Read the model definition and answer for the solid it produces. Units are mm, in the model's axes. Face numbers are marked on the shaded views. A direction names the side the tool comes from. Coordinates: 2 decimals unless noted, no trailing zeros. Loops run counter-clockwise (first coordinate to the right, second up) from the corner with the lowest first, then second, coordinate; pieces in that order, holes last. Notation, with made-up numbers: M 33.5,21 L 51.5,21 A8 ccw 51.5,36 Z; hole C -2.75,28.5 d8. An arc over 180 degrees is marked long. One line per item, written item: value. Start each with the question number.
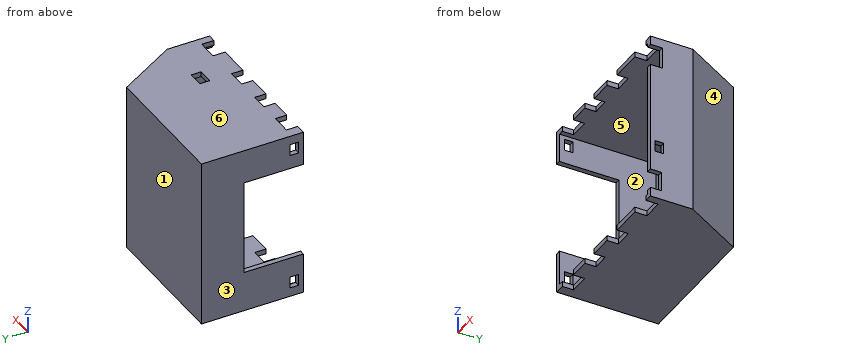
```python
from build123d import *

# Parameters (mm, degrees)
BOSS_EXTRUDE1_DEPTH = 100
SHELL1_T            = -3
SKETCH2_W           = 56.015644735
SKETCH2_H           = 35
CUT_EXTRUDE1_DEPTH  = 10
SKETCH3_W           = 12.606592538
SKETCH3_H           = 6.980178381
SKETCH3_W_2         = 11.515112664
SKETCH3_H_2         = 6.37986445
CUT_EXTRUDE2_DEPTH  = 10
SKETCH4_W           = 9.169229256
SKETCH4_H           = 5.894504522
CUT_EXTRUDE3_DEPTH  = 10
SKETCH5_W           = 6.776014824
SKETCH5_H           = 5.054240566
CUT_EXTRUDE4_DEPTH  = 10
SKETCH6_W           = 11.990530565
SKETCH6_H           = 7.12730724
CUT_EXTRUDE5_DEPTH  = 122.475306133
SKETCH8_W           = 6.563036955
SKETCH8_H           = 5.005706152
CUT_EXTRUDE6_DEPTH  = 10
SKETCH9_W           = 11.789009043
SKETCH9_H           = 6.673883815
SKETCH9_W_2         = 10.731021053
SKETCH9_H_2         = 6.623503435
SKETCH9_W_3         = 9.824174203
SKETCH9_H_3         = 6.573123054
CUT_EXTRUDE7_DEPTH  = 122.475306133


with BuildPart() as part:
    # Sketch1 → Boss-Extrude1 (new body)
    with BuildSketch(Plane.XY):
        Polygon((-50, 12.5), (-50, 47.5), (29.792740578, 47.5), (50, 12.5), (50, -12.5), (-50, -12.5), align=None)
    extrude(amount=BOSS_EXTRUDE1_DEPTH)

    # Shell1
    shell1_openings = [part.faces().sort_by_distance(p)[0] for p in [
        (0, -12.5, 50),
    ]]
    offset(amount=SHELL1_T, openings=shell1_openings, kind=Kind.INTERSECTION)

    # Sketch2 → Cut-Extrude1 (cut)
    with BuildSketch(Plane.ZY.offset(50)):
        with Locations((51.884685058, 5)):
            Rectangle(SKETCH2_W, SKETCH2_H)
    extrude(amount=-CUT_EXTRUDE1_DEPTH, mode=Mode.SUBTRACT)

    # Sketch3 → Cut-Extrude2 (cut)
    with BuildSketch(Plane(origin=(50, 0, 0), x_dir=(0, 0, -1), z_dir=(1, 0, 0))):
        with Locations((-88.542199405, -9.009910809)):
            Rectangle(SKETCH3_W, SKETCH3_H)
        with Locations((-11.156276384, -9.310067775)):
            Rectangle(SKETCH3_W_2, SKETCH3_H_2)
    extrude(amount=-CUT_EXTRUDE2_DEPTH, mode=Mode.SUBTRACT)

    # Sketch4 → Cut-Extrude3 (cut)
    with BuildSketch(Plane.XY.offset(100)):
        with Locations((18.993403459, 9.968133111)):
            Rectangle(SKETCH4_W, SKETCH4_H)
    extrude(amount=-CUT_EXTRUDE3_DEPTH, mode=Mode.SUBTRACT)

    # Sketch5 → Cut-Extrude4 (cut)
    with BuildSketch(Plane.ZY.offset(50)):
        with Locations((8.609898129, -7.132480119)):
            Rectangle(SKETCH5_W, SKETCH5_H)
        with Locations((91.390101871, -7.132480119)):
            Rectangle(SKETCH5_W, SKETCH5_H)
    extrude(amount=-CUT_EXTRUDE4_DEPTH, mode=Mode.SUBTRACT)

    # Sketch6 → Cut-Extrude5 (cut, through all)
    with BuildSketch(Plane.XY.offset(100)):
        with Locations((39.347077193, -8.93634638)):
            Rectangle(SKETCH6_W, SKETCH6_H)
    extrude(amount=-CUT_EXTRUDE5_DEPTH, mode=Mode.SUBTRACT)

    # Sketch8 → Cut-Extrude6 (cut)
    with BuildSketch(Plane(origin=(50, 0, 0), x_dir=(0, 0, -1), z_dir=(1, 0, 0))):
        with Locations((-32.231091097, -7.194817018)):
            Rectangle(SKETCH8_W, SKETCH8_H)
    extrude(amount=-CUT_EXTRUDE6_DEPTH, mode=Mode.SUBTRACT)

    # Sketch9 → Cut-Extrude7 (cut, through all)
    with BuildSketch(Plane.XY.offset(100)):
        with Locations((-38.087567679, -9.163058093)):
            Rectangle(SKETCH9_W, SKETCH9_H)
        with Locations((9.093658686, -9.188248283)):
            Rectangle(SKETCH9_W_2, SKETCH9_H_2)
        with Locations((-15.038543588, -9.213438473)):
            Rectangle(SKETCH9_W_3, SKETCH9_H_3)
    extrude(amount=-CUT_EXTRUDE7_DEPTH, mode=Mode.SUBTRACT)


solid = part.part
```
1) Section D-D (y = -2) is taken. Determine the outline of the cut face in (x, z).
2) A tool of negligible diameter and unlimited length cuts with its end or side. For the marked faces 1 and 2, from which of +Z, -Z, +X, -X, +Y, -Y can it reach the whole face along a straight path? Write none if from no direction.
3) Consider line 1 along Z through (x, y) = (20, 41.5); line 2 along X through (y, z) = (3.5, 11.5); line 3 along Y through (x, z) = (12, 60.5). Determine where each line is inside the solid, lowest interval first.
4) Flat-ended cylindrical pins translate along their axes: pin 1 (2.5 mm diameter, centred on x = -48.5, z = 58.5, fed in from -Y); pin 2 (0.9 mm diameter, centred on x = -12.5, z = 98.5, fed in from -Y); pin 3 (1.5 mm diameter, centred on x = -34, z = 78.5, fed in from -Y); pin 4 (0.9 mm diameter, centred on x = -49, y = 13, fed in from -Z). Find the tip coordinate at first contact, or state that the pin passes through.
5) Section B-B (y = 10) is taken. Determine the outline of the cut face in (x, z), then the cut area to 3 significant figures.
6) Section A-A (z = 32) is taken. Determine the outline of the cut face in (x, y), then the cut area to 3 significant figures.
7) For a pull along X with two mould halves and no side action, classify the marked faces 3, 4, 5 and 6 as released by +X, released by -X, zero draft, split by the parting line, or undercut.
8) Section C-C (x = -23.5) is taken. Determine the outline of the cut face in (y, z), then the cut area to 3 significant figures.
Results found:
1. outline: M -50,0 L 50,0 L 50,100 L -50,100 L -50,79.89 L -47,79.89 L -47,97 L 47,97 L 47,3 L -47,3 L -47,23.88 L -50,23.88 Z
2. face 1: +Z, -Z, +X, -X, +Y
2. face 2: -Y
3. line 1: z = 0 to 3, 97 to 100
3. line 2: x = -50 to -47, 47 to 50
3. line 3: y = 44.5 to 47.5
4. pin 1: stops at y = 22.5
4. pin 2: stops at y = -5.93
4. pin 3: stops at y = 44.5
4. pin 4: stops at z = 0
5. outline: M -50,0 L 50,0 L 50,100 L 23.58,100 L 23.58,97 L 47,97 L 47,3 L -47,3 L -47,23.88 L -50,23.88 Z; M -50,79.89 L -47,79.89 L -47,97 L 14.41,97 L 14.41,100 L -50,100 Z
5. area: 968 mm²
6. outline: M -50,22.5 L -47,22.5 L -47,44.5 L 28.06,44.5 L 47,11.7 L 47,-4.69 L 50,-4.69 L 50,12.5 L 29.79,47.5 L -50,47.5 Z; M 47,-12.5 L 50,-12.5 L 50,-9.7 L 47,-9.7 Z
6. area: 479 mm²
7. face 3: released by -X
7. face 4: released by +X
7. face 5: undercut
7. face 6: zero draft
8. outline: M -12.5,0 L 47.5,0 L 47.5,100 L -12.5,100 L -12.5,97 L 44.5,97 L 44.5,3 L -12.5,3 Z
8. area: 642 mm²
